```python
from build123d import *

# Parameters (mm, degrees)
SKETCH1_W           = 59
SKETCH1_H           = 15.6
BOSS_EXTRUDE1_DEPTH = 19.5
SKETCH2_R           = 3
CUT_EXTRUDE1_DEPTH  = 2
SKETCH3_R           = 3
SKETCH3_R_2         = 2.5
CUT_EXTRUDE2_DEPTH  = 5
SKETCH4_R           = 1.5
CUT_EXTRUDE3_DEPTH  = 65.067230313
CHAMFER1_SIZE       = 0.2


with BuildPart() as part:
    # Sketch1 → Boss-Extrude1 (new body)
    with BuildSketch(Plane.XY):
        with Locations((29.5, 7.8)):
            Rectangle(SKETCH1_W, SKETCH1_H)
    extrude(amount=BOSS_EXTRUDE1_DEPTH)

    # Sketch2 → Cut-Extrude1 (cut)
    with BuildSketch(Plane.ZY):
        with Locations((10.4, 10.7)):
            Circle(SKETCH2_R)
        with Locations((4.5, 4.6)):
            Circle(SKETCH2_R)
    extrude(amount=-CUT_EXTRUDE1_DEPTH, mode=Mode.SUBTRACT)

    # Sketch3 → Cut-Extrude2 (cut)
    with BuildSketch(Plane(origin=(59, 0, 0), x_dir=(0, 0, -1), z_dir=(1, 0, 0))):
        with Locations((-4.5, 10)):
            Circle(SKETCH3_R)
        with Locations((-11.5, 4.4)):
            Circle(SKETCH3_R_2)
    extrude(amount=-CUT_EXTRUDE2_DEPTH, mode=Mode.SUBTRACT)

    # Sketch4 → Cut-Extrude3 (cut, through all)
    with BuildSketch(Plane.XZ):
        with Locations(Location((21.6, 11.5, 0), (0, 0, 270))):
            Circle(SKETCH4_R)
        with Locations(Location((37.4, 11.5, 0), (0, 0, 270))):
            Circle(SKETCH4_R)
    extrude(amount=-CUT_EXTRUDE3_DEPTH, mode=Mode.SUBTRACT)

    # Chamfer1
    chamfer1_edges = [part.edges().sort_by_distance(p)[0] for p in [
        (59, 7.8, 19.5),
        (29.5, 15.6, 19.5),
        (54, 10, 7.5),
        (59, 10, 7.5),
        (59, 4.4, 14),
        (21.6, 15.6, 13),
        (21.6, 0, 13),
        (37.4, 15.6, 13),
        (37.4, 0, 13),
        (0, 7.8, 19.5),
        (29.5, 15.6, 0),
        (59, 7.8, 0),
        (29.5, 0, 0),
        (0, 7.8, 0),
        (0, 15.6, 9.75),
        (59, 15.6, 9.75),
        (59, 0, 9.75),
        (0, 0, 9.75),
        (29.5, 0, 19.5),
    ]]
    chamfer(chamfer1_edges, length=CHAMFER1_SIZE)


solid = part.part
```
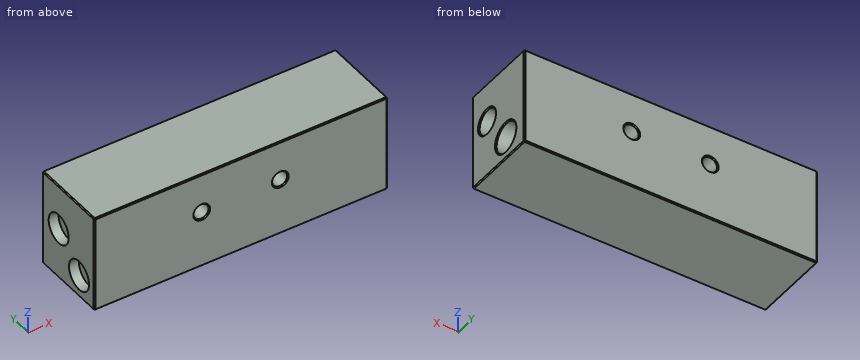
CAD build for the part. Positions are in the model's coordinates, mm. Round coordinates to 2 decimals unless told otherwise and drop trailing zeros. Write each loop counter-clockwise with the first axis right and the second up, starting at its lowest first coordinate (ties: lowest second). Pieces come first, ordered by that corner, then holes. Notation, with made-up numbers: (33, 54) -> (44, 54) arc R8 cw to (44, 68) -> close; hole circle Ø1 at (41.25, 24.25). An arc over 180 degrees is marked (long way). Answer in a Markdown table with one row per item. Add a question column.
Item 1: Saw through at D-D, the plane z = 11.25. Count the separate pieces of the cut face and the enclosed holes in it, then the cut area to 3 significant figures.
Item 2: Saw through at B-B, the plane z = 4.5. Write the cut outline in (x, y).
Item 3: Saw through at A-A, the plane x = 21.6. Write the cut outline in (y, z).
Item 4: Drill centre lines: line 1 (Y direction, x = 55.6, z = 11.5); line 2 (Y direction, x = 0.8, z = 4.5); line 3 (X direction, y = 1.75, z = 5). Where is each one in solid material? Low to high. Write a range as from..to.
Item 5: Drop flat-ended pins along their axis: pin 1 Ø1.8 at (x, z) = (21.6, 11.5) entering from -Y; pin 2 Ø3 at (y, z) = (3.5, 5) entering from -X. Give the stop position or say it passes through.
Item 6: Saw through at C-C, the plane y = 10. Write the cut outline in (x, z), then the cut area to 3 significant figures.
Findings below:
| question | item | result |
|---|---|---|
| 1 | separate pieces | 3 |
| 1 | enclosed holes | 0 |
| 1 | area | 791 mm^2 |
| 2 | outline | (0, 0.2) -> (0.2, 0) -> (58.8, 0) -> (59, 0.2) -> (59, 6.8) -> (58.8, 7) -> (54.2, 7) -> (54, 7.2) -> (54, 12.8) -> (54.2, 13) -> (58.8, 13) -> (59, 13.2) -> (59, 15.4) -> (58.8, 15.6) -> (0.2, 15.6) -> (0, 15.4) -> (0, 7.6) -> (2, 7.6) -> (2, 1.6) -> (0, 1.6) -> close |
| 3 | outline | (0, 0.2) -> (0.2, 0) -> (15.4, 0) -> (15.6, 0.2) -> (15.6, 9.8) -> (15.4, 10) -> (0.2, 10) -> (0, 9.8) -> close; (0, 13.2) -> (0.2, 13) -> (15.4, 13) -> (15.6, 13.2) -> (15.6, 19.3) -> (15.4, 19.5) -> (0.2, 19.5) -> (0, 19.3) -> close |
| 4 | line 1 | y = 0..1.9, 6.9..15.6 |
| 4 | line 2 | y = 0..1.6, 7.6..15.6 |
| 4 | line 3 | x = 2..59 |
| 5 | pin 1 | passes through |
| 5 | pin 2 | stops at x = 2 |
| 6 | outline | (0, 0.2) -> (0.2, 0) -> (58.8, 0) -> (59, 0.2) -> (59, 1.3) -> (58.8, 1.5) -> (54.2, 1.5) -> (54, 1.7) -> (54, 7.3) -> (54.2, 7.5) -> (58.8, 7.5) -> (59, 7.7) -> (59, 19.3) -> (58.8, 19.5) -> (0.2, 19.5) -> (0, 19.3) -> (0, 13.32) -> (2, 13.32) -> (2, 7.48) -> (0, 7.48) -> close; hole circle Ø3 at (21.6, 11.5); hole circle Ø3 at (37.4, 11.5) |
| 6 | area | 1,090 mm^2 |
